Verification items for the finished model (mm, model axes). A direction names the side the tool comes from. Coordinates: 2 decimals unless noted, no trailing zeros. Order: outer loops, then holes, each group sorted by start corner. A loop starts at its lowest first (then second) coordinate and runs counter-clockwise, first axis right, second up. Notation, with made-up numbers: M 50,52.25 L 77,52.25 A15 cw 77,68.25 Z; hole C 76.25,-31.75 d1. An arc over 180 degrees is marked long. Answer as a JSON object with one key per item and string values. Group by question number.
(1) Cross-section at A-A (y = -1.75). Enter the section's corners in (x, z), plus the area to 3 significant figures.
(2) Access from +Z, -Z, +X, -X, +Y, -Y to the whole of each face (thin tool, end or side, straight path). Record for faces 1 (the face through (-2, 1, -0.762)), 2 (the face through (0, 0.762, 0)), 3 (the face through (-1, 0, 2)), 4 (the face through (-0.762, 1, 2)).
(3) Mould release check, pull along X, two halves, no side actions. Record for faces 5 (the face through (-2, 1, 0.762)), 6 (the face through (-0.4, -1.8, -1.8)), 7 (the face through (0.762, 1, -2)): released by +X, released by -X, zero draft, split by the parting line, or undercut.
(4) Gauge pin test, flat ends, axial feed: pin 1 Ø2 at (x, y) = (-2.5, 2) entering from -Z; pin 2 Ø1 at (y, z) = (1.5, -2) entering from -X; pin 3 Ø1.4 at (x, y) = (2, 2) entering from +Z; pin 4 Ø1 at (y, z) = (0, -0.5) entering from -X. Record the tip position at first contact, or that the pin passes through.
(5) Material ranges on line 1 (Y direction, x = -0.75, z = -0.25); line 2 (Z direction, x = -2, y = 1.25); line 3 (X direction, y = 1.25, z = 2.5), recorded low to high.
from build123d import *

# Parameters (mm, degrees)
CUT_EXTRUDE1_DEPTH  = 3.048
SKETCH3_R           = 1.842682312
BOSS_EXTRUDE1_DEPTH = 3.556


with BuildPart() as part:
    # Sketch1 → Revolve1 (revolve)
    with BuildSketch(Plane.XY):
        with BuildLine():
            Line((0, 0), (3.683, 0))
            ThreePointArc((3.683, 0), (2.367551224, 2.032774275), (0, 2.54))
            Line((0, 2.54), (0, 0))
        make_face()
    revolve(axis=Axis((0, 23.833116883, 0), (0, -1, 0)))

    # Sketch2 → Cut-Extrude1 (cut)
    with BuildSketch(Plane(origin=(0, 3.81, 0), x_dir=(-1, 0, 0), z_dir=(0, -1, 0))):
        Polygon((-0.762, -0.762), (-0.762, -3.958262237), (0.762, -3.958262237), (0.762, -0.762), (5.504133478, -0.762), (5.504133478, 0.762), (0.762, 0.762), (0.762, 3.972126553), (-0.762, 3.972126553), (-0.762, 0.762), (-5.060475364, 0.762), (-5.060475364, -0.762), align=None)
    extrude(amount=CUT_EXTRUDE1_DEPTH, mode=Mode.SUBTRACT)

    # Sketch3 → Boss-Extrude1 (add)
    with BuildSketch(Plane.XZ):
        Circle(SKETCH3_R)
    extrude(amount=BOSS_EXTRUDE1_DEPTH)


solid = part.part
Taken from the geometry:
{
 "1": {"outline": "C 0,0 d3.69", "area": "10.7 mm²"},
 "2": {"face 1": "+X, -X, +Y", "face 2": "+Y", "face 3": "-Y", "face 4": "+Z, -Z, +Y"},
 "3": {"face 5": "zero draft", "face 6": "split by the parting line", "face 7": "undercut"},
 "4": {"pin 1": "stops at z = -2.57", "pin 2": "stops at x = -2.78", "pin 3": "stops at z = 2.57", "pin 4": "stops at x = -3.68"},
 "5": {"line 1": "y = -3.56 to 0.76", "line 2": "z = -2.44 to -0.76, 0.76 to 2.44", "line 3": "x = -1.93 to -0.76, 0.76 to 1.93"}
}
